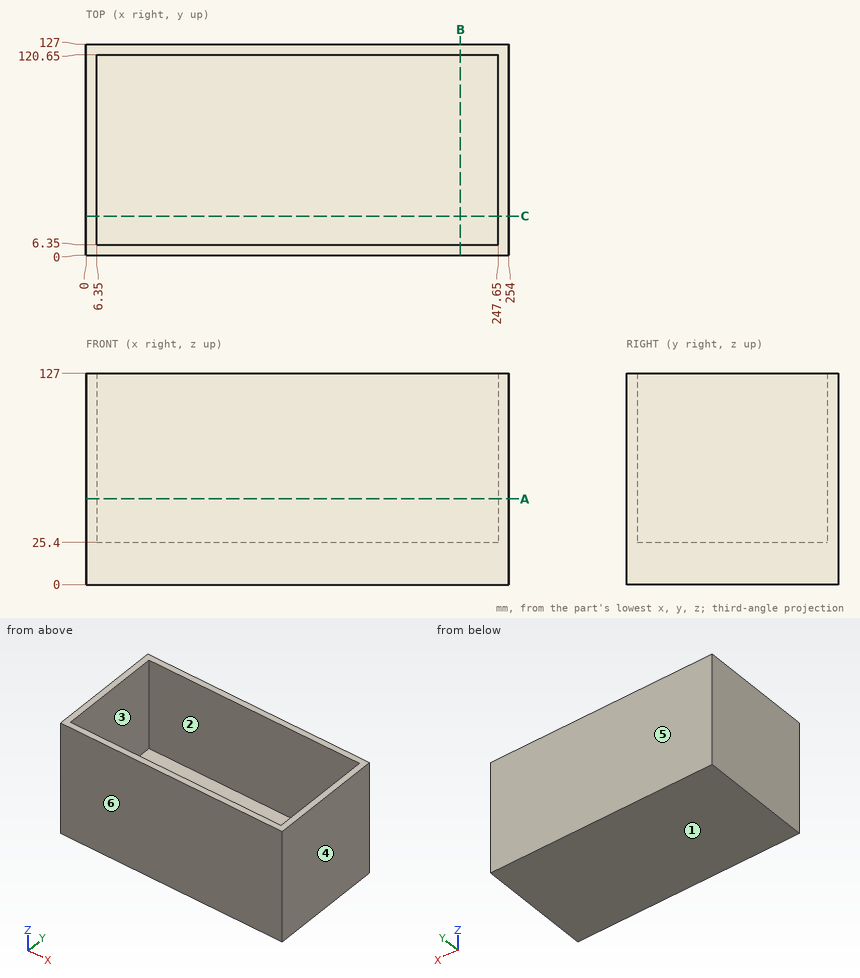
Study the drawing (mm; zero at the part's minimum x, y, z) and answer. A direction names the side the tool comes from. Give positions to 0.01 mm unless a question says otherwise; leave off trailing zeros. Order: outer loops, then holes, each group sorted by start corner. A loop starts at its lowest first (then second) coordinate and runs counter-clockwise, first axis right, second up. Notation, with made-up numbers: (-33, 70.5) - (-20, 70.5) arc R15 ccw to (-20, 92.5) - close; hole circle Ø10 at (62, 1). An arc over 180 degrees is marked (long way). Use one line per item in the form item = value. Start each with the question number.
(1) The mould has two halves that part along Y. Classify the marked faces 3, 4, 5 and 6: released by +Y, released by -Y, zero draft, split by the parting line, or undercut.
(2) For the marked faces 1 and 2, determine the directions among +Z, -Z, +X, -X, +Y, -Y from which every point of the face is accessible in a straight line to the end or side of a thin tool.
(3) A cutting plane is placed at C-C, the plane y = 23.5. Write down the section's boundary in (x, z).
(4) A cutting plane is placed at A-A, the plane z = 51.5. Write down the section's boundary in (x, y), then the cut area to 3 significant figures.
(5) A flat-ended cylindrical pin translates along its axis: pin 1 Ø4 at (x, y) = (96.5, 86) entering from +Z. Find the tip coordinate at first contact, or state that the pin passes through.
(6) Consider line 1 (X direction, y = 62.5, z = 63); line 2 (Y direction, x = 56, z = 67.5); line 3 (Z direction, x = 240.5, y = 78.5). Determine where each line is inside the solid, lowest interval first. Write a range as from..to.
(7) A cutting plane is placed at B-B, the plane x = 225. Write down the section's boundary in (y, z), then the cut area to 3 significant figures.
Ans:
q1.face_3 = undercut
q1.face_4 = zero draft
q1.face_5 = released by +Y
q1.face_6 = released by -Y
q2.face_1 = -Z, +X, -X, +Y, -Y
q2.face_2 = +Z
q3.outline = (0, 0) - (254, 0) - (254, 127) - (247.65, 127) - (247.65, 25.4) - (6.35, 25.4) - (6.35, 127) - (0, 127) - close
q4.outline = (0, 0) - (254, 0) - (254, 127) - (0, 127) - close; hole (6.35, 6.35) - (247.65, 6.35) - (247.65, 120.65) - (6.35, 120.65) - close
q4.area = 4,680 mm^2
q5.pin_1 = 25.4
q6.line_1 = 0..6.35, 247.65..254
q6.line_2 = 0..6.35, 120.65..127
q6.line_3 = 0..25.4
q7.outline = (0, 0) - (127, 0) - (127, 127) - (120.65, 127) - (120.65, 25.4) - (6.35, 25.4) - (6.35, 127) - (0, 127) - close
q7.area = 4,520 mm^2
